Source: CAD feature listing. Evaluate the final solid. Frame: model axes, mm. A direction names the side the tool comes from. Give positions to 0.01 mm unless a question says otherwise; leave off trailing zeros. Order: outer loops, then holes, each group sorted by start corner. A loop starts at its lowest first (then second) coordinate and runs counter-clockwise, first axis right, second up. Notation, with made-up numbers: M 54,40.25 L 110,40.25 A30 ccw 110,62.25 Z; hole C 89,36.5 d4. An arc over 180 degrees is marked long. Answer in a Markdown table with one row per item. Add a question column.
(1) Pin query (flat end, axial travel): P1, Ø6, axis at x = 19, z = -5.5, coming from the -Y side; P2, Ø5, axis at y = 35, z = -22, coming from the -X side (3 decimals). Return the tip coordinate at first contact, or that it passes through.
(2) Section query C-C, the plane y = 36.5. Return loops of the section in (x, z), plus the area to 3 significant figures.
(3) Section query A-A, the plane y = 45. Return loops of the section in (x, z), plus the area to 3 significant figures.
(4) Section query B-B, the plane x = 88.9. Return loops of the section in (y, z).
(5) Section query D-D, the plane z = -5.75. Return loops of the section in (x, y), plus the area to 3 significant figures.
(6) Mould query, pull axis Y, two halves, no side actions, for faces 1 (the face through (75, 37, -23.812)), 2 (the face through (3.62, 29.22, -24.6)), 3 (the face through (7.705, 38.32, -24.595)). Classes: pulls with the +Y half, pulls with the -Y half, needs draft (parallel to the pull), parting line crosses it, or undercut.
(7) Material intervals for line 1 along Z through (x, y) = (21, 41.5); line 2 along Y through (x, z) = (12.7, -24.15); line 3 along Y through (x, z) = (88.9, -1.05), sorted ascending.
(8) Set-up query: faces 4 (the face through (75, 49.212, -13)), 5 (the face through (7.705, 38.32, -0.783)). Return all of +Z, -Z, +X, -X, +Y, -Y with unobstructed straight access to the full face (end or side cutting, diameter ignored); none if empty.
from build123d import *

# Parameters (mm, degrees)
SKETCH1_W           = 25.4
SKETCH1_H           = 50.8
SKETCH1_W_2         = 22.225
SKETCH1_H_2         = 47.625
BOSS_EXTRUDE1_DEPTH = 152.4
SKETCH2_R           = 5
SKETCH2_R_2         = 3
CUT_EXTRUDE1_DEPTH  = 152.4


with BuildPart() as part:
    # Sketch1 → Boss-Extrude1 (new body)
    with BuildSketch(Plane(origin=(0, 0, 0), x_dir=(0, 0, -1), z_dir=(1, 0, 0))):
        with Locations((12.7, 25.4)):
            Rectangle(SKETCH1_W, SKETCH1_H)
        with Locations((12.7, 25.4)):
            Rectangle(SKETCH1_W_2, SKETCH1_H_2, mode=Mode.SUBTRACT)
    extrude(amount=BOSS_EXTRUDE1_DEPTH)

    # Sketch2 → Cut-Extrude1 (cut)
    with BuildSketch(Plane.XY):
        with Locations((12.7, 38.1)):
            Circle(SKETCH2_R)
        with Locations((88.9, 38.1)):
            Circle(SKETCH2_R_2)
        with BuildLine():
            Line((12.7, 25.4), (152.4, 25.4))
            Line((152.4, 25.4), (152.4, 0))
            Line((152.4, 0), (0, 0))
            Line((0, 0), (0, 38.1))
            ThreePointArc((0, 38.1), (3.719743879, 29.119743879), (12.7, 25.4))
        make_face()
    extrude(amount=-CUT_EXTRUDE1_DEPTH, mode=Mode.SUBTRACT)


solid = part.part
Values follow:
| question | item | result |
|---|---|---|
| 1 | P1 | stops at y = 49.21 |
| 1 | P2 | stops at x = 0.075 |
| 2 | outline | M 0.1,-25.4 L 7.96,-25.4 L 7.96,-23.81 L 0.1,-23.81 Z; M 0.1,-1.59 L 7.96,-1.59 L 7.96,0 L 0.1,0 Z; M 17.44,-25.4 L 86.36,-25.4 L 86.36,-23.81 L 17.44,-23.81 Z; M 17.44,-1.59 L 86.36,-1.59 L 86.36,0 L 17.44,0 Z; M 91.44,-25.4 L 152.4,-25.4 L 152.4,-23.81 L 91.44,-23.81 Z; M 91.44,-1.59 L 152.4,-1.59 L 152.4,0 L 91.44,0 Z |
| 2 | area | 437 mm² |
| 3 | outline | M 0,-25.4 L 152.4,-25.4 L 152.4,-23.81 L 0,-23.81 Z; M 0,-1.59 L 152.4,-1.59 L 152.4,0 L 0,0 Z |
| 3 | area | 484 mm² |
| 4 | outline | M 25.4,-25.4 L 35.1,-25.4 L 35.1,-23.81 L 25.4,-23.81 Z; M 25.4,-1.59 L 35.1,-1.59 L 35.1,0 L 25.4,0 Z; M 41.1,-25.4 L 50.8,-25.4 L 50.8,0 L 41.1,0 L 41.1,-1.59 L 49.21,-1.59 L 49.21,-23.81 L 41.1,-23.81 Z |
| 5 | outline | M 0,49.21 L 152.4,49.21 L 152.4,50.8 L 0,50.8 Z |
| 5 | area | 242 mm² |
| 6 | face 1 | needs draft |
| 6 | face 2 | pulls with the -Y half |
| 6 | face 3 | undercut |
| 7 | line 1 | z = -25.4 to -23.81, -1.59 to 0 |
| 7 | line 2 | y = 25.4 to 33.1, 43.1 to 50.8 |
| 7 | line 3 | y = 25.4 to 35.1, 41.1 to 50.8 |
| 8 | face 4 | +X, -X, -Y |
| 8 | face 5 | +Z, -Z |
